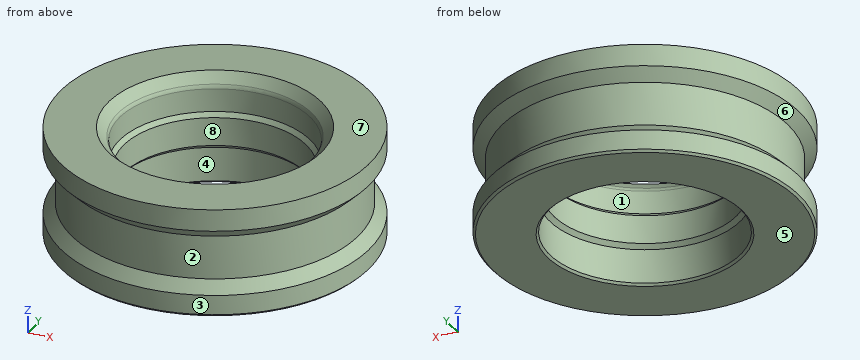
```python
from build123d import *

# Parameters (mm, degrees)
F2_SIZE = 1
F3_R    = 0.5
F4_SIZE = 0.2


with BuildPart() as f1:
    # F0 (on Front) → F1 (revolve)
    with BuildSketch(Plane.XZ):
        Polygon((-8.35, -1.3), (-8.35, 0), (-8.35, 1.3), (-8.725, 1.675), (-8.725, 5), (-14.1, 5), (-14.1, 3), (-13.1, 2), (-13.1, 0), (-13.1, -2), (-14.1, -3), (-14.1, -5), (-8.725, -5), (-8.725, -1.675), align=None)
    revolve(axis=Axis((0, 0, 7.7657741494), (0, 0, 1)))

    # F2
    f2_edges = [f1.edges().sort_by_distance(p)[0] for p in [
        (8.725, 0, 5),
    ]]
    chamfer(f2_edges, length=F2_SIZE)

    # F3
    f3_edges = [f1.edges().sort_by_distance(p)[0] for p in [
        (8.725, 0, 4),
    ]]
    fillet(f3_edges, radius=F3_R)

    # F4
    f4_edges = [f1.edges().sort_by_distance(p)[0] for p in [
        (14.1, 0, -5),
        (8.725, 0, -5),
    ]]
    chamfer(f4_edges, length=F4_SIZE)


solid = f1.part
```
Build history of the part. All positions in model axes, mm. Face numbers are marked on the shaded views. A direction names the side the tool comes from. Round coordinates to 2 decimals unless told otherwise and drop trailing zeros. Write each loop counter-clockwise with the first axis right and the second up, starting at its lowest first coordinate (ties: lowest second). Pieces come first, ordered by that corner, then holes. Notation, with made-up numbers: (21, 27) - (72, 27) arc R23 ccw to (72, 44) - close; hole circle Ø7 at (88.5, 6). An arc over 180 degrees is marked (long way). Answer as CSV lines item,"result".
Q1. Pull direction Z, two halves, no side cores. Call the marked faces 6, 7 and 8: +Z half, -Z half, draft (parallel to the pull), parting line (faces both ways), or undercut.
Report:
face 6,"undercut"
face 7,"+Z half"
face 8,"draft"
Q2. Drop flat-ended pins along their axis: pin 1 (6 mm diameter, centred on x = 7.5, z = -2, fed in from +Y); pin 2 (1 mm diameter, centred on x = 8, z = 0.5, fed in from -Y); pin 3 (3 mm diameter, centred on x = -9.5, z = 3.5, fed in from -Y). Give the stop position or say it passes through.
Report:
pin 1,"stops at y = 13.3"
pin 2,"stops at y = -10.74"
pin 3,"stops at y = -11.61"
Q3. Cut at A-A (z = 0.75). Write the cut outline in (x, y), and give its area (3 significant figures).
Report:
outline,"circle Ø26.2 at (0, 0); hole circle Ø16.7 at (0, 0)"
area,"320 mm^2"
Q4. Drill centre lines: probe 1 along X at (y, z) = (0, -0.65); probe 2 along Y at (x, z) = (-0.25, 3.25). Where is each one in solid material? Low to high. Write a range as [from, to].
Report:
probe 1,"x = [-13.1, -8.35], [8.35, 13.1]"
probe 2,"y = [-14.1, -8.72], [8.72, 14.1]"
Q5. Tool access for the marked faces 1, 2, 3, 4 and 5: list every direction of +Z, -Z, +X, -X, +Y, -Y with a clear straight run to the whole face (end or side of a thin tool).
Report:
face 1,"+Z"
face 2,"none"
face 3,"+Z, -Z"
face 4,"-Z"
face 5,"-Z, +X, -X, +Y, -Y"
